Input: part model. Units: mm. Frame: model coordinates. A direction names the side the tool comes from. Round coordinates to 2 decimals unless told otherwise and drop trailing zeros. Loops run counter-clockwise (first coordinate to the right, second up) from the corner with the lowest first, then second, coordinate; pieces in that order, holes last.
(1) Draft query along X for faces 4 (the face through (10, -6, 0)), 5 (the face through (-0.596, -4.19, -2.685)), 6 (the face through (-5, 0, 0)). Return one class per face: released by +X, released by -X, zero draft, split by the parting line, or undercut.
(2) Cut plane C-C, the plane x = -22. Output: boundary loops of the cut face in (y, z).
(3) Access query for faces 1 (the face through (-19.5, -2, 0)), 2 (the face through (5.96, -12.01, 1.88)), 3 (the face through (-10, -6, -10)). Directions: +Z, -Z, +X, -X, +Y, -Y. A direction counts if a zero-diameter tool reaches every point of the face in a straight line with its end or side. Return the directions, or none.
(4) First-contact query: pin 1 Ø10 at (x, z) = (1, -5) entering from -Y; pin 2 Ø4 at (x, z) = (2, 3) entering from -Y; pin 3 Ø4 at (y, z) = (-3.5, 1.5) entering from -X. Flat tips, straight axial feed; report the tip coordinate or a pass-through.
(5) Cut plane B-B, the plane y = -10. Output: boundary loops of the cut face in (x, z), and give its area (3 significant figures).
(6) Line query: line 1 (Y direction, x = -20.5, z = 5); line 2 (Z direction, x = -1, y = -6.75); line 3 (Z direction, x = -1, y = -9.75). Output: solid intervals per line, ascending.
(7) Cut plane A-A, the plane z = 0. Output: boundary loops of the cut face in (x, y), and give its area (3 significant figures).
from build123d import *

# Parameters (mm, degrees)
F0_R     = 2.75
F1_DEPTH = 5
F2_R     = 2.75
F3_DEPTH = 8
F4_R     = 6.25
F5_DEPTH = 2
F6_SIZE  = 2.5


with BuildPart() as f1:
    # F0 (on Front) → F1 (new body)
    with BuildSketch(Plane.XZ):
        with BuildLine():
            ThreePointArc((0, -10), (10, 0), (0, 10))
            Line((0, 10), (-19.5, 10))
            Line((-19.5, 10), (-19.5, -10))
            Line((-19.5, -10), (0, -10))
        make_face()
        Circle(F0_R, mode=Mode.SUBTRACT)
    extrude(amount=F1_DEPTH)

    # F2 (on face) → F3 (join)
    with BuildSketch(Plane.XZ.offset(5)):
        with BuildLine():
            ThreePointArc((0, -10), (10, 0), (0, 10))
            Line((0, 10), (-19.5, 10))
            ThreePointArc((-19.5, 10), (-29.5, 0), (-19.5, -10))
            Line((-19.5, -10), (0, -10))
        make_face()
        Circle(F2_R, mode=Mode.SUBTRACT)
    extrude(amount=F3_DEPTH)

    # F4 (on face) → F5 (cut)
    with BuildSketch(Plane.XZ.offset(13)):
        Circle(F4_R)
    extrude(amount=-F5_DEPTH, mode=Mode.SUBTRACT)

    # F6
    f6_edges = [f1.edges().sort_by_distance(p)[0] for p in [
        (-2.75, -11, 0),
    ]]
    chamfer(f6_edges, length=F6_SIZE)


solid = f1.part
Reported:
1. face 4: released by +X
1. face 5: undercut
1. face 6: zero draft
2. outline: (-13, -9.68) - (-5, -9.68) - (-5, 9.68) - (-13, 9.68) - close
3. face 1: +Z, -Z, -X, +Y
3. face 2: -Y
3. face 3: -Z, +X, -X, +Y, -Y
4. pin 1: stops at y = -13
4. pin 2: stops at y = -11
4. pin 3: stops at x = -29.5
5. outline: (-19.5, -10) - (0, -10) arc R10 ccw to (0, 10) - (-19.5, 10) arc R10 ccw to start; hole circle Ø8.5 at (0, 0)
5. area: 647 mm2
6. line 1: y = -13 to -5
6. line 2: z = -10 to -2.56, 2.56 to 10
6. line 3: z = -10 to -3.87, 3.87 to 10
7. outline: (-29.5, -13) - (-6.25, -13) - (-6.25, -11) - (-5.25, -11) - (-2.75, -8.5) - (-2.75, 0) - (-19.5, 0) - (-19.5, -5) - (-29.5, -5) - close; (2.75, -8.5) - (5.25, -11) - (6.25, -11) - (6.25, -13) - (10, -13) - (10, 0) - (2.75, 0) - close
7. area: 372 mm2
